Check sheet for the modelled part. Datum: model origin and axes. Units: mm. Round coordinates to 2 decimals unless told otherwise and drop trailing zeros. Loops run counter-clockwise (first coordinate to the right, second up) from the corner with the lowest first, then second, coordinate; pieces in that order, holes last. Notation, with made-up numbers: M 52,52 L 64,52 A23 cw 64,71 Z; hole C 35.5,-29.5 d5. An arc over 180 degrees is marked long. Write item = value, one per line. Start each with the question number.
(1) Scan lines: L1, parallel to Y at x = 0, z = 1.4; L2, parallel to Y at x = 32, z = 2.4; L3, parallel to Y at x = -31, z = 0.4. Record each from-to range of solid material in increasing order. Write a range as from..to.
(2) Go/stop test with flat-tipped pins: P1, Ø4, axis at x = -22.56, y = -46.85, coming from the +Z side; P2, Ø1, axis at x = 36, z = 2, coming from the +Y side. Record where each tip stops, or that it passes through.
(3) Cross-section at C-C on z = 1.65. State how many separate pieces and enclosed holes the cut face has, plus the area to 3 significant figures.
(4) Cross-section at B-B on y = 52. Record the boundary of the cut face in (x, z).
(5) Cross-section at D-D on x = 47.5. Record the boundary of the cut face in (y, z).
(6) Cross-section at A-A on x = 0. Record the boundary of the cut face in (y, z), plus the area to 3 significant figures.
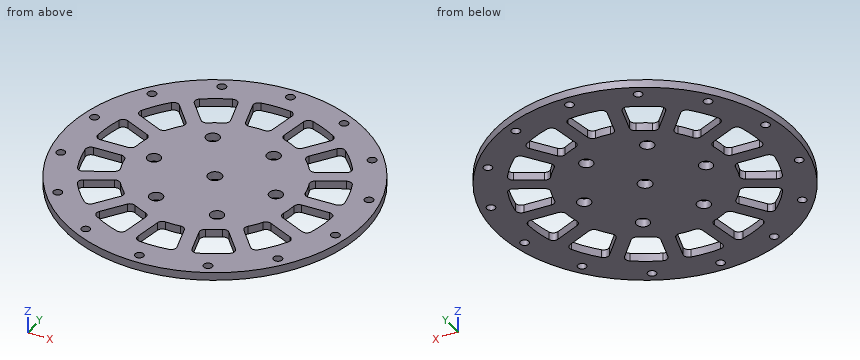
from build123d import *

# Parameters (mm, degrees)
SKETCH_1_R          = 56
SKETCH_1_R_2        = 1.6
SKETCH_1_R_3        = 2.6
SKETCH_1_R_4        = 2.5
EXTRUDE_1_DEPTH     = 3
SKETCH_2_R          = 45
SKETCH_2_R_2        = 31
CUT_EXTRUDE_1_DEPTH = 10
EXTRUDE_1_2_DEPTH   = 3
FILLET_2_R          = 2


with BuildPart() as part:
    # Sketch 1 → Extrude 1 (new body)
    with BuildSketch(Plane.XY):
        Circle(SKETCH_1_R)
        with Locations((0, 52)):
            Circle(SKETCH_1_R_2, mode=Mode.SUBTRACT)
        with Locations((22.561954434, 46.850381131)):
            Circle(SKETCH_1_R_2, mode=Mode.SUBTRACT)
        with Locations((40.655237088, 32.421469697)):
            Circle(SKETCH_1_R_2, mode=Mode.SUBTRACT)
        with Locations((50.696251433, 11.571088566)):
            Circle(SKETCH_1_R_2, mode=Mode.SUBTRACT)
        with Locations((50.696251433, -11.571088566)):
            Circle(SKETCH_1_R_2, mode=Mode.SUBTRACT)
        with Locations((40.655237088, -32.421469697)):
            Circle(SKETCH_1_R_2, mode=Mode.SUBTRACT)
        with Locations((22.561954434, -46.850381131)):
            Circle(SKETCH_1_R_2, mode=Mode.SUBTRACT)
        with Locations((0, -52)):
            Circle(SKETCH_1_R_2, mode=Mode.SUBTRACT)
        with Locations((-22.561954434, -46.850381131)):
            Circle(SKETCH_1_R_2, mode=Mode.SUBTRACT)
        with Locations((-40.655237088, -32.421469697)):
            Circle(SKETCH_1_R_2, mode=Mode.SUBTRACT)
        with Locations((-50.696251433, -11.571088566)):
            Circle(SKETCH_1_R_2, mode=Mode.SUBTRACT)
        with Locations((-50.696251433, 11.571088566)):
            Circle(SKETCH_1_R_2, mode=Mode.SUBTRACT)
        with Locations((-40.655237088, 32.421469697)):
            Circle(SKETCH_1_R_2, mode=Mode.SUBTRACT)
        with Locations((-22.561954434, 46.850381131)):
            Circle(SKETCH_1_R_2, mode=Mode.SUBTRACT)
        Circle(SKETCH_1_R_3, mode=Mode.SUBTRACT)
        with Locations((11.25, 19.485571585)):
            Circle(SKETCH_1_R_4, mode=Mode.SUBTRACT)
        with Locations((-11.25, 19.485571585)):
            Circle(SKETCH_1_R_4, mode=Mode.SUBTRACT)
        with Locations((-22.5, 0)):
            Circle(SKETCH_1_R_4, mode=Mode.SUBTRACT)
        with Locations((-11.25, -19.485571585)):
            Circle(SKETCH_1_R_4, mode=Mode.SUBTRACT)
        with Locations((11.25, -19.485571585)):
            Circle(SKETCH_1_R_4, mode=Mode.SUBTRACT)
        with Locations((22.5, 0)):
            Circle(SKETCH_1_R_4, mode=Mode.SUBTRACT)
    extrude(amount=EXTRUDE_1_DEPTH)

    # Sketch 2 → Cut-Extrude 1 (cut)
    with BuildSketch(Plane.XY.offset(3)):
        Circle(SKETCH_2_R)
        Circle(SKETCH_2_R_2, mode=Mode.SUBTRACT)
    extrude(amount=-CUT_EXTRUDE_1_DEPTH, mode=Mode.SUBTRACT)


with BuildPart() as cut_extrude_1_piece_1:
    # of the separate pieces the step leaves, piece 1, a body of its own (cut_extrude_1_pieces)
    add(part.part.solids().sort_by_distance((56, 0, 0))[0])



with BuildPart() as cut_extrude_1_piece_2:
    # of the separate pieces the step leaves, piece 2, a body of its own (cut_extrude_1_pieces)
    add(part.part.solids().sort_by_distance((31, 0, 0))[0])


with BuildPart() as cut_extrude_1_piece_1_1:
    add(cut_extrude_1_piece_1.part)

    add(cut_extrude_1_piece_2.part)  # Extrude 1 2 merges Cut-Extrude 1 piece 2
    # Sketch 3 → Extrude 1 2 (add)
    with BuildSketch(Plane.XY.offset(3)):
        Polygon((-14.609298387, 45.373678206), (-9.303630073, 25.350616171), (-4.470429278, 26.631307419), (-9.776097591, 46.654369454), align=None)
        Polygon((6.524378129, 47.219008495), (2.616939079, 26.876809755), (7.527173635, 25.933625467), (11.434612685, 46.275824207), align=None)
        Polygon((26.36582154, 39.71203505), (14.019191351, 23.079721546), (18.033927495, 20.099470936), (30.380557684, 36.731784439), align=None)
        Polygon((40.98519064, 24.339606026), (22.644770843, 14.71141143), (24.968840842, 10.284369682), (43.309260639, 19.912564278), align=None)
        Polygon((47.486940083, 4.146419523), (26.785275749, 3.429325856), (26.958369039, -1.567677117), (47.660033372, -0.85058345), align=None)
        Polygon((44.583318653, -16.868016219), (25.620628293, -8.531979761), (23.608461624, -13.109226236), (42.571151984, -21.445262694), align=None)
        Polygon((32.849424186, -34.541534476), (19.381501187, -18.803422148), (15.582608846, -22.054332325), (29.050531844, -37.792444653), align=None)
        Polygon((14.609298387, -45.373678206), (9.303630073, -25.350616171), (4.470429278, -26.631307419), (9.776097591, -46.654369454), align=None)
        Polygon((-6.524378129, -47.219008495), (-2.616939079, -26.876809755), (-7.527173635, -25.933625467), (-11.434612685, -46.275824207), align=None)
        Polygon((-26.36582154, -39.71203505), (-14.019191351, -23.079721546), (-18.033927495, -20.099470936), (-30.380557684, -36.731784439), align=None)
        Polygon((-40.98519064, -24.339606026), (-22.644770843, -14.71141143), (-24.968840842, -10.284369682), (-43.309260639, -19.912564278), align=None)
        Polygon((-47.486940083, -4.146419523), (-26.785275749, -3.429325856), (-26.958369039, 1.567677117), (-47.660033372, 0.85058345), align=None)
        Polygon((-44.583318653, 16.868016219), (-25.620628293, 8.531979761), (-23.608461624, 13.109226236), (-42.571151984, 21.445262694), align=None)
        Polygon((-32.849424186, 34.541534476), (-19.381501187, 18.803422148), (-15.582608846, 22.054332325), (-29.050531844, 37.792444653), align=None)
    extrude(amount=-EXTRUDE_1_2_DEPTH)

    # Fillet 2
    fillet_2_edges = [cut_extrude_1_piece_1_1.edges().sort_by_distance(p)[0] for p in [
        (16.410002001, 26.300415098, 1.5),
        (20.424738144, 23.320164488, 1.5),
        (28.788199205, 34.586696669, 1.5),
        (24.773463062, 37.56694728, 1.5),
        (40.943876522, 18.670805429, 1.5),
        (28.520293368, 12.148780442, 1.5),
        (26.196223368, 16.57582219, 1.5),
        (38.619806522, 23.097847177, 1.5),
        (44.990116949, -0.943067809, 1.5),
        (30.967054712, -1.428818566, 1.5),
        (30.793961422, 3.568184407, 1.5),
        (44.817023659, 4.053935164, 1.5),
        (40.125512947, -20.370154902, 1.5),
        (27.280411084, -14.723422534, 1.5),
        (29.292577753, -10.146176058, 1.5),
        (42.137679616, -15.792908426, 1.5),
        (6.020431416, 44.595452745, 1.5),
        (10.930665972, 43.652268457, 1.5),
        (27.313558999, -35.762682992, 1.5),
        (18.190547469, -25.101872097, 1.5),
        (21.98943981, -21.85096192, 1.5),
        (31.11245134, -32.511772815, 1.5),
        (9.091819712, -44.071973116, 1.5),
        (5.497822835, -30.508588038, 1.5),
        (10.33102363, -29.22789679, 1.5),
        (13.925020507, -42.791281868, 1.5),
        (-10.930665972, -43.652268457, 1.5),
        (-8.283813038, -29.872703955, 1.5),
        (-3.373578481, -30.815888243, 1.5),
        (-6.020431416, -44.595452745, 1.5),
        (-28.788199205, -34.586696669, 1.5),
        (-20.424738144, -23.320164488, 1.5),
        (-16.410002001, -26.300415098, 1.5),
        (-24.773463062, -37.56694728, 1.5),
        (-40.943876522, -18.670805429, 1.5),
        (-28.520293368, -12.148780442, 1.5),
        (-26.196223368, -16.57582219, 1.5),
        (-38.619806522, -23.097847177, 1.5),
        (-44.990116949, 0.943067809, 1.5),
        (-30.967054712, 1.428818566, 1.5),
        (-30.793961422, -3.568184407, 1.5),
        (-44.817023659, -4.053935164, 1.5),
        (3.373578481, 30.815888243, 1.5),
        (-40.125512947, 20.370154902, 1.5),
        (-27.280411084, 14.723422534, 1.5),
        (-29.292577753, 10.146176058, 1.5),
        (-42.137679616, 15.792908426, 1.5),
        (-27.313558999, 35.762682992, 1.5),
        (-18.190547469, 25.101872097, 1.5),
        (-21.98943981, 21.85096192, 1.5),
        (-31.11245134, 32.511772815, 1.5),
        (8.283813038, 29.872703955, 1.5),
        (-10.33102363, 29.22789679, 1.5),
        (-5.497822835, 30.508588038, 1.5),
        (-9.091819712, 44.071973116, 1.5),
        (-13.925020507, 42.791281868, 1.5),
    ]]
    fillet(fillet_2_edges, radius=FILLET_2_R)


solid = cut_extrude_1_piece_1_1.part
Result:
q1.L1 = -56..-53.6, -50.4..-45, -31..-2.6, 2.6..31, 45..50.4, 53.6..56
q1.L2 = -45.96..-31.41, -16.8..-11.34, -1.54..3.7, 13.98..19.62, 31.64..45.96
q1.L3 = -46.64..-32.62, -19.1..-13.45, -4.32..2.55, 10.9..16.36, 31.55..46.64
q2.P1 = 3
q2.P2 = 43.31
q3.separate_pieces = 1
q3.enclosed_holes = 35
q3.area = 7,290 mm^2
q4.outline = M -20.78,0 L -1.6,0 L -1.6,3 L -20.78,3 Z; M 1.6,0 L 20.78,0 L 20.78,3 L 1.6,3 Z
q5.outline = M -29.66,0 L 29.66,0 L 29.66,3 L -29.66,3 Z
q6.outline = M -56,0 L -53.6,0 L -53.6,3 L -56,3 Z; M -50.4,0 L -45,0 L -45,3 L -50.4,3 Z; M -31,0 L -2.6,0 L -2.6,3 L -31,3 Z; M 2.6,0 L 31,0 L 31,3 L 2.6,3 Z; M 45,0 L 50.4,0 L 50.4,3 L 45,3 Z; M 53.6,0 L 56,0 L 56,3 L 53.6,3 Z
q6.area = 217 mm^2
